Job drawing, mm, ordinate dimensions from the low corner. One solid piece. A direction names the side the tool comes from. Round coordinates to 2 decimals unless told otherwise and drop trailing zeros. Order: outer loops, then holes, each group sorted by start corner. A loop starts at its lowest first (then second) coordinate and runs counter-clockwise, first axis right, second up. Notation, with made-up numbers: (45, 55.25) - (66, 55.25) arc R23 ccw to (66, 76.25) - close; hole circle Ø10 at (36.5, -35.75). An arc over 180 degrees is marked (long way). Write each question's results on one line, items separated by ' | '. Start each with the question number.
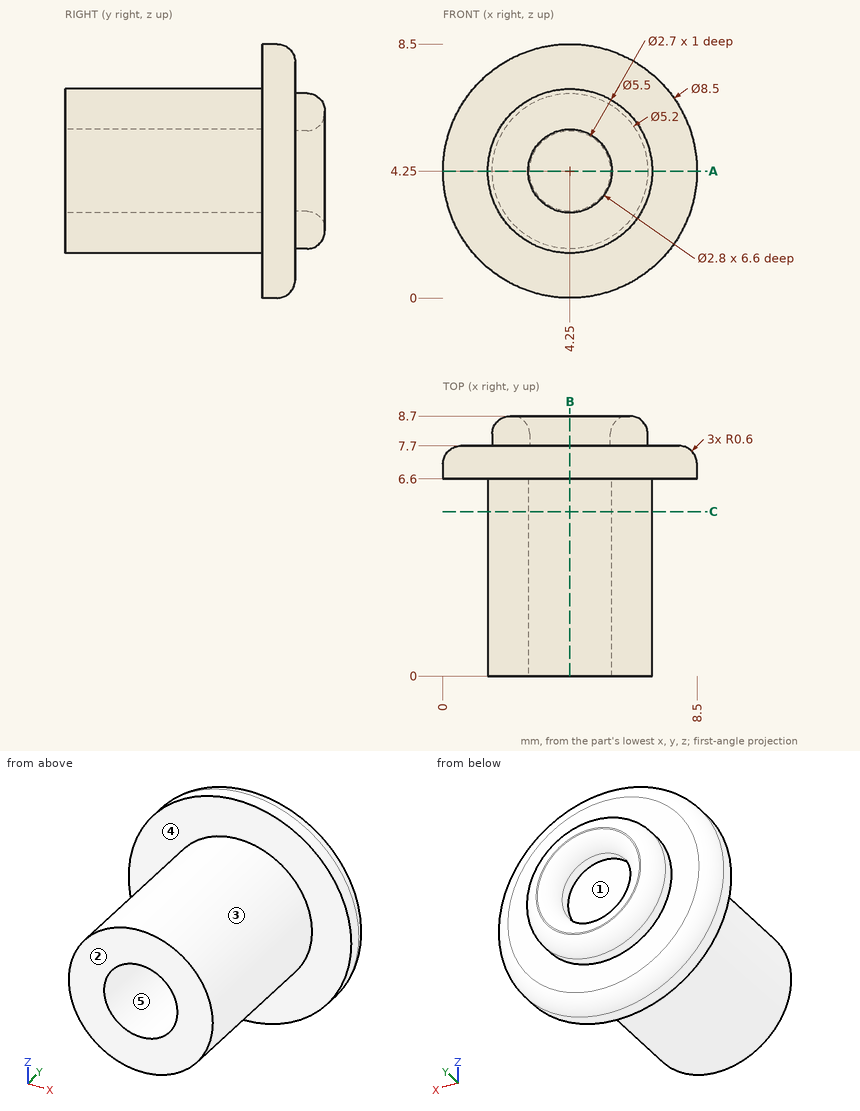
1. Cut at A-A (z = 4.25). List the corners of the cut face in (x, y).
2. 3-axis set-ups, long thin cutter, end or side, ignore diameter. For the marked faces 1 and 2: which of +Z, -Z, +X, -X, +Y, -Y reach the whole face in a straight line?
3. Mould opens along X. For the marked faces 3, 4 and 5 say: pulls with the +X half, pulls with the -X half, needs draft (parallel to the pull), parting line crosses it, or undercut.
4. Wall check: line 1 (X direction, y = 5, z = 4.25); line 2 (X direction, y = 7.9, z = 4.25). Give the ranges that are in metal, low to high. Write a range as from..to.
5. Flat gauge pins, fed straight in: pin 1 Ø1.5 at (y, z) = (2, 2.5) entering from +X; pin 2 Ø2 at (x, z) = (5, 5.5) entering from +Y; pin 3 Ø4 at (x, y) = (2.5, 2) entering from +Z; pin 4 Ø1.5 at (x, y) = (2.5, 1.5) entering from +Z. Where does each tip first touch, or does it go through?
6. Cut at C-C (y = 5.5). List the corners of the cut face in (x, z).
7. Cut at B-B (x = 4.25). List the corners of the cut face in (y, z), plus the area to 3 significant figures.
A:
1) outline: (0, 6.6) - (1.5, 6.6) - (1.5, 0) - (2.85, 0) - (2.85, 6.6) - (5.65, 6.6) - (5.65, 0) - (7, 0) - (7, 6.6) - (8.5, 6.6) - (8.5, 7.1) arc R0.6 ccw to (7.9, 7.7) - (6.85, 7.7) - (6.85, 8.1) arc R0.6 ccw to (6.25, 8.7) - (6.2, 8.7) arc R0.6 ccw to (5.6, 8.1) - (5.6, 7.7) - (2.9, 7.7) - (2.9, 8.1) arc R0.6 ccw to (2.3, 8.7) - (2.25, 8.7) arc R0.6 ccw to (1.65, 8.1) - (1.65, 7.7) - (0.6, 7.7) arc R0.6 ccw to (0, 7.1) - close
2) face 1: +Y | face 2: +Z, -Z, +X, -X, -Y
3) face 3: parting line crosses it | face 4: needs draft | face 5: undercut
4) line 1: x = 1.5..2.85, 5.65..7 | line 2: x = 1.65..2.9, 5.6..6.85
5) pin 1: stops at x = 6.81 | pin 2: stops at y = 8.7 | pin 3: stops at z = 7 | pin 4: stops at z = 6.81
6) outline: circle Ø5.5 at (4.25, 4.25); hole circle Ø2.8 at (4.25, 4.25)
7) outline: (0, 1.5) - (6.6, 1.5) - (6.6, 0) - (7.1, 0) arc R0.6 ccw to (7.7, 0.6) - (7.7, 1.65) - (8.1, 1.65) arc R0.6 ccw to (8.7, 2.25) - (8.7, 2.3) arc R0.6 ccw to (8.1, 2.9) - (7.7, 2.9) - (7.7, 5.6) - (8.1, 5.6) arc R0.6 ccw to (8.7, 6.2) - (8.7, 6.25) arc R0.6 ccw to (8.1, 6.85) - (7.7, 6.85) - (7.7, 7.9) arc R0.6 ccw to (7.1, 8.5) - (6.6, 8.5) - (6.6, 7) - (0, 7) - (0, 5.65) - (6.6, 5.65) - (6.6, 2.85) - (0, 2.85) - close | area: 29.2 mm^2
